Geometry: final body of the model. Coordinates: model frame, mm. Face numbers are marked on the shaded views. A direction names the side the tool comes from. Coordinates: 2 decimals unless noted, no trailing zeros. Loops run counter-clockwise (first coordinate to the right, second up) from the corner with the lowest first, then second, coordinate; pieces in that order, holes last. Notation, with made-up numbers: (2.25, -30) - (16.25, -30) arc R16 cw to (16.25, -7) - close; hole circle Ø5 at (-14.5, 67.25). An arc over 180 degrees is marked (long way). Return JSON: item names as keys, results as strings.
from build123d import *

# Parameters (mm, degrees)
SKETCH_W        = 100
SKETCH_H        = 64
SKETCH_R        = 5
SKETCH_R_2      = 3.2
SKETCH_R_3      = 4
PAD_DEPTH       = 15
SKETCH001_R     = 11.02
POCKET_DEPTH    = 7.2
SKETCH002_R     = 6
POCKET001_DEPTH = 7
SKETCH003_R     = 3.2
POCKET002_DEPTH = 15
FILLET_R        = 2


with BuildPart() as part:
    # Sketch → Pad (new body)
    with BuildSketch(Plane.XY):
        with Locations((50, 32)):
            Rectangle(SKETCH_W, SKETCH_H)
        with Locations((50, 42.85)):
            Circle(SKETCH_R, mode=Mode.SUBTRACT)
        with Locations((20, 10)):
            Circle(SKETCH_R_2, mode=Mode.SUBTRACT)
        with Locations((80, 10)):
            Circle(SKETCH_R_2, mode=Mode.SUBTRACT)
        with Locations((82, 42.85)):
            Circle(SKETCH_R_3, mode=Mode.SUBTRACT)
        with Locations((18, 42.85)):
            Circle(SKETCH_R_3, mode=Mode.SUBTRACT)
    extrude(amount=PAD_DEPTH)

    # Sketch001 (on Face11 of Pad) → Pocket (cut)
    with BuildSketch(Plane.XY.offset(15)):
        with Locations((50, 42.85)):
            Circle(SKETCH001_R)
    extrude(amount=-POCKET_DEPTH, mode=Mode.SUBTRACT)

    # Sketch002 (on Face4 of Pocket) → Pocket001 (cut)
    with BuildSketch(Plane(origin=(0, 0, 0), x_dir=(1, 0, 0), z_dir=(0, 0, -1))):
        with Locations((20, -10)):
            Circle(SKETCH002_R)
        with Locations((80, -10)):
            Circle(SKETCH002_R)
        with Locations((40, -10)):
            Circle(SKETCH002_R)
        with Locations((60, -10)):
            Circle(SKETCH002_R)
    extrude(amount=-POCKET001_DEPTH, mode=Mode.SUBTRACT)

    # Sketch003 (on Face5 of Pocket001) → Pocket002 (cut)
    with BuildSketch(Plane.XY.offset(15)):
        with Locations((40, 10)):
            Circle(SKETCH003_R)
        with Locations((60, 10)):
            Circle(SKETCH003_R)
    extrude(amount=-POCKET002_DEPTH, mode=Mode.SUBTRACT)

    # Fillet
    fillet_edges = [part.edges().sort_by_distance(p)[0] for p in [
        (0, 64, 7.5),
        (100, 64, 7.5),
        (0, 0, 7.5),
        (100, 0, 7.5),
    ]]
    fillet(fillet_edges, radius=FILLET_R)


solid = part.part
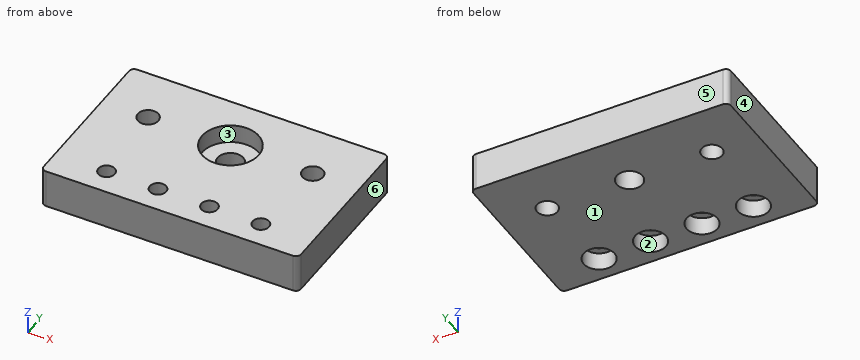
Item 1: Mould query, pull axis X, two halves, no side actions, for the marked faces 3, 4, 5 and 6. Classes: +X half, -X half, draft (parallel to the pull), parting line (faces both ways), or undercut.
Worked out:
{"face 3": "undercut", "face 4": "-X half", "face 5": "draft", "face 6": "+X half"}
Item 2: Section query A-A, the plane z = 4.75. Return loops of the section in (x, y), and give its area (3 significant figures).
Worked out:
{"outline": "(0, 2) arc R2 ccw to (2, 0) - (98, 0) arc R2 ccw to (100, 2) - (100, 62) arc R2 ccw to (98, 64) - (2, 64) arc R2 ccw to (0, 62) - close; hole circle Ø12 at (20, 10); hole circle Ø8 at (18, 42.85); hole circle Ø12 at (40, 10); hole circle Ø10 at (50, 42.85); hole circle Ø12 at (60, 10); hole circle Ø12 at (80, 10); hole circle Ø8 at (82, 42.85)", "area": "5,770 mm^2"}
Item 3: Section query D-D, the plane x = 18. Return loops of the section in (y, z).
Worked out:
{"outline": "(0, 0) - (4.34, 0) - (4.34, 7) - (7.5, 7) - (7.5, 15) - (0, 15) - close; (12.5, 7) - (15.66, 7) - (15.66, 0) - (38.85, 0) - (38.85, 15) - (12.5, 15) - close; (46.85, 0) - (64, 0) - (64, 15) - (46.85, 15) - close"}
Item 4: Section query B-B, the plane y = 42.85. Return loops of the section in (x, z).
Worked out:
{"outline": "(0, 0) - (14, 0) - (14, 15) - (0, 15) - close; (22, 0) - (45, 0) - (45, 7.8) - (38.98, 7.8) - (38.98, 15) - (22, 15) - close; (55, 0) - (78, 0) - (78, 15) - (61.02, 15) - (61.02, 7.8) - (55, 7.8) - close; (86, 0) - (100, 0) - (100, 15) - (86, 15) - close"}
Item 5: Reachability of the marked faces 1 and 2 from +Z, -Z, +X, -X, +Y, -Y: full face, straight path, thin tool, end or side. Return the list, or none.
Worked out:
{"face 1": "-Z, +X, -X, +Y, -Y", "face 2": "-Z"}
Item 6: Ray query, probe 1 along X at (y, z) = (10, 4); probe 2 along Y at (x, z) = (60, 4.5); probe 3 along X at (y, z) = (6.5, 3). Return the intervals inside material, ascending. Write a range as from..to.
Worked out:
{"probe 1": "0..14, 26..34, 46..54, 66..74, 86..100", "probe 2": "0..4, 16..64", "probe 3": "0..15.13, 24.87..35.13, 44.87..55.13, 64.87..75.13, 84.87..100"}
Item 7: Section query C-C, the plane x = 50. Return loops of the section in (y, z), and give its area (3 significant figures).
Worked out:
{"outline": "(0, 0) - (37.85, 0) - (37.85, 7.8) - (31.83, 7.8) - (31.83, 15) - (0, 15) - close; (47.85, 0) - (64, 0) - (64, 15) - (53.87, 15) - (53.87, 7.8) - (47.85, 7.8) - close", "area": "723 mm^2"}
Item 8: First-contact query: pin 1 Ø8 at (x, y) = (50, 42.85) entering from -Z; pin 2 Ø11 at (x, y) = (20, 10) entering from -Z. Flat tips, straight axial feed; report the tip coordinate or a pass-through.
Worked out:
{"pin 1": "through", "pin 2": "z = 7"}
